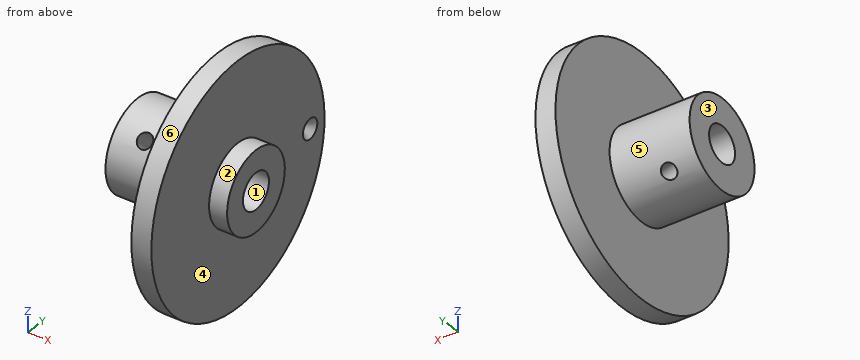
from build123d import *

# Parameters (mm, degrees)
ESQUISSE4_R             = 3.7
ENL_V_MAT_EXTRU_2_DEPTH = 25


with BuildPart() as part:
    # Esquisse1 → Base-Révolution (revolve)
    with BuildSketch(Plane.XY, mode=Mode.PRIVATE) as base_r_volution_sk:
        Polygon((0, 9), (59, 9), (59, 20), (50, 20), (50, 60), (40, 60), (40, 22.5), (0, 22.5), align=None)
    revolve(base_r_volution_sk.sketch.rotate(Axis((-20, 0, 0), (1, 0, 0)), 90), axis=Axis((-20, 0, 0), (1, 0, 0)))

    # Esquisse2 → Enlèvement de matière-Révolution1 (revolve, cut)
    with BuildSketch(Plane.XY, mode=Mode.PRIVATE) as enl_vement_de_mati_re_r_volution1_sk:
        Polygon((45, 50), (50, 55), (50, 50), align=None)
    revolve(enl_vement_de_mati_re_r_volution1_sk.sketch.rotate(Axis((21.308708687, 50, 0), (1, 0, 0)), 270), axis=Axis((21.308708687, 50, 0), (1, 0, 0)), mode=Mode.SUBTRACT)

    # Esquisse4 → Enlèv. mat.-Extru.2 (cut, symmetric)
    with BuildSketch(Plane(origin=(0, 0, 0), x_dir=(1, 0, 0), z_dir=(0, -0.7071067811865488, 0.7071067811865462))):
        with Locations(Location((15, 0, 0), (0, 0, 270))):
            Circle(ESQUISSE4_R)
    extrude(amount=ENL_V_MAT_EXTRU_2_DEPTH, both=True, mode=Mode.SUBTRACT)


solid = part.part
Model file for the job. Use its own axes, mm. Face numbers are marked on the shaded views. A direction names the side the tool comes from. Give positions to 0.01 mm unless a question says otherwise; leave off trailing zeros. Write each loop counter-clockwise with the first axis right and the second up, starting at its lowest first coordinate (ties: lowest second). Pieces come first, ordered by that corner, then holes. Notation, with made-up numbers: (8, 79.25) - (28, 79.25) arc R35 cw to (28, 115.25) - close; hole circle Ø9 at (39, 24.25). An arc over 180 degrees is marked (long way). Answer as CSV lines item,"result".
1. Band-saw the part on B-B (x = 47.5). Write the cut outline in (y, z).
Responses:
outline,"circle Ø120 at (0, 0); hole circle Ø18 at (0, 0); hole circle Ø5 at (50, 0)"
2. Band-saw the part on D-D (y = -45). Write the cut outline in (x, z), and give its area (3 significant figures).
Responses:
outline,"(40, -39.69) - (50, -39.69) - (50, 39.69) - (40, 39.69) - close"
area,"794 mm2"
3. Pin check, flat tips, straight feed: pin 1 (1.5 mm diameter, centred on y = 43.5, z = 15, fed in from +X); pin 2 (5 mm diameter, centred on x = 41.5, z = 2.5, fed in from +Y); pin 3 (3 mm diameter, centred on x = 9, z = 7.5, fed in from -Y); pin 4 (16 mm diameter, centred on y = 0, z = 0, fed in from +X). Stop position of each tip, or through.
Responses:
pin 1,"stops at x = 50"
pin 2,"stops at y = 60"
pin 3,"stops at y = -21.69"
pin 4,"passes through"
4. Drill centre lines: L1, parallel to Y at x = 44, z = 0; L2, parallel to Y at x = 20, z = 0; L3, parallel to X at y = -31.5, z = 45. Where is each one in solid material? Low to high. Write a range as [from, to].
Responses:
L1,"y = [-60, -9], [9, 60]"
L2,"y = [-22.5, -9], [9, 22.5]"
L3,"x = [40, 50]"
5. Band-saw the part on C-C (z = 35). Write the cut outline in (x, y), and give its area (3 significant figures).
Responses:
outline,"(40, -48.73) - (50, -48.73) - (50, 48.73) - (40, 48.73) - close"
area,"975 mm2"
6. Band-saw the part on A-A (y = 0). Write the cut outline in (x, z), and give its area (3 significant figures).
Responses:
outline,"(0, -22.5) - (40, -22.5) - (40, -60) - (50, -60) - (50, -20) - (59, -20) - (59, -9) - (0, -9) - close; (0, 9) - (59, 9) - (59, 20) - (50, 20) - (50, 60) - (40, 60) - (40, 22.5) - (0, 22.5) - close"
area,"2,300 mm2"
7. 3-axis set-ups, long thin cutter, end or side, ignore diameter. For the marked faces 4, 5 and 6: which of +Z, -Z, +X, -X, +Y, -Y reach the whole face in a straight line?
Responses:
face 4,"+X"
face 5,"-X"
face 6,"+X, -X"
8. Two-plate mould, pull along Y, no slides. Class the marked faces 1, 2 and 3: +Y half, -Y half, draft (parallel to the pull), parting line (faces both ways), or undercut.
Responses:
face 1,"undercut"
face 2,"parting line"
face 3,"draft"
